The model under review builds one solid part; all positions refer to its coordinate system, in mm. A direction names the side the tool comes from. Coordinates: 2 decimals unless noted, no trailing zeros. Write each loop counter-clockwise with the first axis right and the second up, starting at its lowest first coordinate (ties: lowest second). Pieces come first, ordered by that corner, then holes. Notation, with made-up numbers: (-35, 58) - (-9, 58) arc R16 ccw to (-9, 72) - close; hole circle Ø11 at (-5, -3.5). An arc over 180 degrees is marked (long way). Put each result on its own line as item: value.
from build123d import *

# Parameters (mm, degrees)
F0_R          = 9.5
F1_DEPTH      = 8.5
F1_DEPTH_BACK = 10.8
F2_R          = 11
F3_DEPTH      = 2.5
F6_DEPTH      = 3
F7_R          = 7
F8_DEPTH      = 5.5


with BuildPart() as f1:
    # F0 (on Top) → F1 (new body, two sides)
    with BuildSketch(Plane.XY) as f1_sk:
        Circle(F0_R)
    extrude(amount=F1_DEPTH)
    extrude(f1_sk.sketch, amount=-F1_DEPTH_BACK)

    # F2 (on Top) → F3 (join)
    with BuildSketch(Plane.XY):
        Circle(F2_R)
    extrude(amount=F3_DEPTH)

    # F5 (on offset) → F6 (join)
    with BuildSketch(Plane.XY.offset(-3)):
        with BuildLine():
            Line((10.136474, 6.73394), (0.763526, 12.145414))
            ThreePointArc((0.763526, 12.145414), (0, 12.35), (-0.763526, 12.145414))
            Line((-0.763526, 12.145414), (-10.136474, 6.73394))
            ThreePointArc((-10.136474, 6.73394), (-10.695414, 6.175), (-10.9, 5.411474))
            Line((-10.9, 5.411474), (-10.9, -5.411474))
            ThreePointArc((-10.9, -5.411474), (-10.695414, -6.175), (-10.136474, -6.73394))
            Line((-10.136474, -6.73394), (-0.763526, -12.145414))
            ThreePointArc((-0.763526, -12.145414), (0, -12.35), (0.763526, -12.145414))
            Line((0.763526, -12.145414), (10.136474, -6.73394))
            ThreePointArc((10.136474, -6.73394), (10.695414, -6.175), (10.9, -5.411474))
            Line((10.9, -5.411474), (10.9, 5.411474))
            ThreePointArc((10.9, 5.411474), (10.695414, 6.175), (10.136474, 6.73394))
        make_face()
    extrude(amount=-F6_DEPTH)

    # F7 (on face) → F8 (join)
    with BuildSketch(Plane(origin=(0, 0, -10.8), x_dir=(1, 0, 0), z_dir=(0, 0, -1))):
        Circle(F7_R)
    extrude(amount=F8_DEPTH)


solid = f1.part
1. Consider section C-C on y = -3.5. State the section outline as (x, z) points.
Determined:
outline: (-10.9, -6) - (-8.83, -6) - (-8.83, -10.8) - (-6.06, -10.8) - (-6.06, -16.3) - (6.06, -16.3) - (6.06, -10.8) - (8.83, -10.8) - (8.83, -6) - (10.9, -6) - (10.9, -3) - (8.83, -3) - (8.83, 0) - (10.43, 0) - (10.43, 2.5) - (8.83, 2.5) - (8.83, 8.5) - (-8.83, 8.5) - (-8.83, 2.5) - (-10.43, 2.5) - (-10.43, 0) - (-8.83, 0) - (-8.83, -3) - (-10.9, -3) - close
2. Machinability: for faces 1 (the cylindrical face through (4.38, -8.43, -1.48)), 2 (the cylindrical face through (6.466, 2.681, -13.512)), 3 (the flat face through (5.38, -9.48, -4.48)), 4 (the flat face through (5.52, 9.4, -4.48)), which of the approach directions +Z, -Z, +X, -X, +Y, -Y give a long, thin tool a straight path to every point of the face, cutting with its end or side? Answer none if there is none.
Determined:
face 1: none
face 2: -Z
face 3: -Z, +X, -Y
face 4: -Z, +X, +Y
3. To check wall thickness, follow probe 1 along Z at (x, y) = (3.5, -10.5); probe 2 along Z at (x, y) = (9.25, 1.25); probe 3 along Z at (x, y) = (-10, -2.75). State the ranges of each line that lie inside material, in increasing order.
Determined:
probe 1: z = -6 to -3
probe 2: z = -10.8 to 8.5
probe 3: z = -6 to -3, 0 to 2.5
4. Consider section B-B on z = -3.75. State the section outline as (x, y) points, plus the area to 3 significant figures.
Determined:
outline: (-10.9, -5.41) arc R1.53 ccw to (-10.14, -6.73) - (-0.76, -12.15) arc R1.53 ccw to (0.76, -12.15) - (10.14, -6.73) arc R1.53 ccw to (10.9, -5.41) - (10.9, 5.41) arc R1.53 ccw to (10.14, 6.73) - (0.76, 12.15) arc R1.53 ccw to (-0.76, 12.15) - (-10.14, 6.73) arc R1.53 ccw to (-10.9, 5.41) - close
area: 411 mm^2
5. The part is to be moulded in two halves that separate along Z. For faces 5 (the flat face through (0, 0, -16.3)), 6 (the flat face through (-10, 0, 0)), 7 (the flat face through (-5.52, -9.4, -4.48)), say which applies: +Z half, -Z half, draft (parallel to the pull), parting line (faces both ways), or undercut.
Determined:
face 5: -Z half
face 6: undercut
face 7: draft
6. Consider section A-A on x = 0. State the section outline as (y, z) points, plus the area to 3 significant figures.
Determined:
outline: (-12.35, -6) - (-9.5, -6) - (-9.5, -10.8) - (-7, -10.8) - (-7, -16.3) - (7, -16.3) - (7, -10.8) - (9.5, -10.8) - (9.5, -6) - (12.35, -6) - (12.35, -3) - (9.5, -3) - (9.5, 0) - (11, 0) - (11, 2.5) - (9.5, 2.5) - (9.5, 8.5) - (-9.5, 8.5) - (-9.5, 2.5) - (-11, 2.5) - (-11, 0) - (-9.5, 0) - (-9.5, -3) - (-12.35, -3) - close
area: 468 mm^2
7. For pin 1 Ø3 at (x, z) = (7, 3.5) entering from -Y; pin 2 Ø3.5 at (y, z) = (-0.5, -4) entering from -X; pin 3 Ø4 at (y, z) = (3.5, -1.5) entering from +X, all flat-tipped, find the tip position at first contact; note any pin that passes through.
Determined:
pin 1: stops at y = -9.3
pin 2: stops at x = -10.9
pin 3: stops at x = 10.9
8. Consider section D-D on y = -8.75. State the section outline as (x, z) points, plus the area to 3 significant figures.
Determined:
outline: (-6.67, 0) - (-3.7, 0) - (-3.7, -3) - (-6.64, -3) - (-6.64, -6) - (-3.7, -6) - (-3.7, -10.8) - (3.7, -10.8) - (3.7, -6) - (6.64, -6) - (6.64, -3) - (3.7, -3) - (3.7, 0) - (6.67, 0) - (6.67, 2.5) - (3.7, 2.5) - (3.7, 8.5) - (-3.7, 8.5) - (-3.7, 2.5) - (-6.67, 2.5) - close
area: 175 mm^2
